from build123d import *

# Parameters (mm, degrees)
SKETCH2_W                                      = 19.05
SKETCH2_H                                      = 31.75
BOSS_EXTRUDE1_DEPTH                            = 3.175
CUT_EXTRUDE1_DEPTH                             = 23.857707289
SKETCH6_W                                      = 1.27
SKETCH6_H                                      = 17.78
SKETCH6_H_2                                    = 1.27
SKETCH6_W_2                                    = 3.81
CUT_EXTRUDE2_DEPTH                             = 23.857707289
CBORE_FOR_4_SOCKET_HEAD_CAP_SCREW1_D           = 3.2639
CBORE_FOR_4_SOCKET_HEAD_CAP_SCREW1_DEPTH       = 5.08
CBORE_FOR_4_SOCKET_HEAD_CAP_SCREW1_CBORE_D     = 5.55752
CBORE_FOR_4_SOCKET_HEAD_CAP_SCREW1_CBORE_DEPTH = 2.8448
F_4_40_TAPPED_HOLE1_D                          = 2.2606
SKETCH20_W                                     = 12.7
SKETCH20_H                                     = 6.35
BOSS_EXTRUDE2_DEPTH                            = 6.35
SKETCH21_W                                     = 6.35
SKETCH21_H                                     = 12.7
BOSS_EXTRUDE4_DEPTH                            = 6.35
SKETCH22_R                                     = 1.5875
CUT_EXTRUDE3_DEPTH                             = 33.065928179


with BuildPart() as part:
    # Sketch2 → Boss-Extrude1 (new, symmetric)
    with BuildSketch(Plane.XY):
        Rectangle(SKETCH2_W, SKETCH2_H)
    extrude(amount=BOSS_EXTRUDE1_DEPTH, both=True)

    # Sketch4 → Cut-Extrude1 (cut, through all)
    with BuildSketch(Plane(origin=(-1.506852909, 3.110534069, 3.175), x_dir=(1, 0, 0), z_dir=(0, 0, 1))):
        Polygon((-8.018147091, 12.764465931), (-8.018147091, 10.224465931), (-1.668147091, 10.224465931), (-1.668147091, 2.604465931), (4.681852909, 2.604465931), (4.681852909, 10.224465931), (11.031852909, 10.224465931), (11.031852909, 12.764465931), align=None)
    extrude(amount=-CUT_EXTRUDE1_DEPTH, mode=Mode.SUBTRACT)

    # Sketch6 → Cut-Extrude2 (cut, through all)
    with BuildSketch(Plane(origin=(-1.506852909, 3.110534069, 3.175), x_dir=(1, 0, 0), z_dir=(0, 0, 1))):
        with Locations((5.316852909, 0.064465931)):
            Rectangle(SKETCH6_W, SKETCH6_H)
        with Locations((5.316852909, -9.460534069)):
            Rectangle(SKETCH6_W, SKETCH6_H_2)
        with Locations((7.856852909, -9.460534069)):
            Rectangle(SKETCH6_W_2, SKETCH6_H_2)
    extrude(amount=-CUT_EXTRUDE2_DEPTH, mode=Mode.SUBTRACT)

    # CBORE for #4 Socket Head Cap Screw1
    with Locations(Plane(origin=(9.525, 0, 0), x_dir=(0, 0, -1), z_dir=(1, 0, 0))):
        with Locations((0, 0.9525)):
            CounterBoreHole(CBORE_FOR_4_SOCKET_HEAD_CAP_SCREW1_D / 2, CBORE_FOR_4_SOCKET_HEAD_CAP_SCREW1_CBORE_D / 2, CBORE_FOR_4_SOCKET_HEAD_CAP_SCREW1_CBORE_DEPTH, depth=CBORE_FOR_4_SOCKET_HEAD_CAP_SCREW1_DEPTH)

    # #4-40 Tapped Hole1 (through all)
    with Locations(Plane(origin=(3.175, 0, 0), x_dir=(0, 0, -1), z_dir=(1, 0, 0))):
        with Locations((0, 0.9525)):
            Hole(F_4_40_TAPPED_HOLE1_D / 2)

    # Sketch20 → Boss-Extrude2 (add, through all)
    with BuildSketch(Plane.XY.offset(3.175)):
        with Locations((15.875, -12.7)):
            Rectangle(SKETCH20_W, SKETCH20_H)
    boss_extrude2 = extrude(amount=-BOSS_EXTRUDE2_DEPTH)

    # Mirror1: Boss-Extrude2 across plane
    add(boss_extrude2.mirror(Plane(origin=(0, 0, 0), x_dir=(0, 0, 1), z_dir=(1, 0, 0))))

    # Sketch21 → Boss-Extrude4 (add, through all)
    with BuildSketch(Plane(origin=(0, 0, -3.175), x_dir=(-1, 0, 0), z_dir=(0, 0, -1))):
        with Locations((0, -15.875)):
            Rectangle(SKETCH21_W, SKETCH21_H)
    extrude(amount=-BOSS_EXTRUDE4_DEPTH)

    # Sketch22 → Cut-Extrude3 (cut, through all)
    with BuildSketch(Plane(origin=(0, 0, -3.175), x_dir=(-1, 0, 0), z_dir=(0, 0, -1))):
        with Locations((0, -19.05)):
            Circle(SKETCH22_R)
    extrude(amount=-CUT_EXTRUDE3_DEPTH, mode=Mode.SUBTRACT)


solid = part.part
Work out the finished part from the listing and answer in its coordinate system (mm). A direction names the side the tool comes from. Coordinates: 2 decimals unless noted, no trailing zeros. Write each loop counter-clockwise with the first axis right and the second up, starting at its lowest first coordinate (ties: lowest second). Pieces come first, ordered by that corner, then holes. Notation, with made-up numbers: M 34.25,-18.75 L 70.25,-18.75 A25 cw 70.25,3.25 Z; hole C 23,42.5 d7. An arc over 180 degrees is marked long. Use one line per item in the form item = value. Start each with the question number.
1. A tool of negligible diameter and unlimited length cuts with its end or side. For faces 5 (the face through (3.175, -1, 0)), 6 (the face through (3.175, -19, 0)), 7 (the face through (6.68, 1, -2)), 8 (the face through (-13, -15.875, 0)), from which of +Z, -Z, +X, -X, +Y, -Y can it reach the whole face along a straight path? Write none if from no direction.
2. The part is cut by section B-B (x = 0). Give the vertices of the cut face in (y, z) (1 decimal), plus the area to 3 significant figures.
3. Each of these flat-tipped pins is pushed along its axis until it touches: P1, Ø1.9, axis at y = -20, z = 1.5, coming from the -X side (3 decimals); P2, Ø1.9, axis at x = 15.5, z = 0, coming from the +Y side (3 decimals); P3, Ø1.9, axis at x = 17.5, z = -0.5, coming from the -Y side (3 decimals). Where does it stop, or does it pass through?
4. The part is cut by section C-C (z = 0). Give the number of separate pieces and of enclosed holes in the cut face, plus the area to 3 significant figures.
5. The part is cut by section A-A (y = -3.5). Give the vertices of the cut face in (x, z) (3 decimals).
6. The part is cut by section D-D (x = 18.5). Give the vertices of the cut face in (y, z) (3 decimals), plus the area to 3 significant figures.
7. Straight lines are drawn through the part: probe 1 along Y at (x, z) = (8, 0) (3 decimals); probe 2 along Y at (x, z) = (5.4, 0) (3 decimals); probe 3 along X at (y, z) = (4, 2.75) (3 decimals). For each, find the intervals that lie inside material, in ascending order. Write a range as from..to.
8. The mould has two halves that part along X. Classify faces 1 (the face through (8.255, -6, 0)), 2 (the face through (-22.225, -13, 0)), 3 (the face through (0, -6, 3.175)), 4 (the face through (-3.175, 10, 0)): released by +X, released by -X, zero draft, split by the parting line, or undercut.
Evaluation:
q1.face_5 = +Z, -Z
q1.face_6 = +Z, -Z, +X, -Y
q1.face_7 = +X
q1.face_8 = +Z, -Z, -X, -Y
q2.outline = M -22.2,-3.2 L -20.6,-3.2 L -20.6,3.2 L -22.2,3.2 Z; M -17.5,-3.2 L 5.7,-3.2 L 5.7,3.2 L -17.5,3.2 Z; hole C 1,0 d2.3
q2.area = 153 mm^2
q3.P1 = -3.175
q3.P2 = -9.525
q3.P3 = -15.875
q4.separate_pieces = 3
q4.enclosed_holes = 1
q4.area = 621 mm^2
q5.outline = M -9.525,-3.175 L 3.175,-3.175 L 3.175,3.175 L -9.525,3.175 Z; M 4.445,-3.175 L 9.525,-3.175 L 9.525,3.175 L 4.445,3.175 Z
q6.outline = M -15.875,-3.175 L -9.525,-3.175 L -9.525,3.175 L -15.875,3.175 Z
q6.area = 40.3 mm^2
q7.probe_1 = -15.875..-6.985, -5.715..-1.826, 3.731..13.335
q7.probe_2 = -15.875..-6.985, -5.715..-0.679, 2.584..13.335
q7.probe_3 = -9.525..3.175, 4.445..9.525
q8.face_1 = undercut
q8.face_2 = released by -X
q8.face_3 = zero draft
q8.face_4 = undercut
